Read the model definition and answer for the solid it produces. Units are mm, in the model's axes. A direction names the side the tool comes from. Coordinates: 2 decimals unless noted, no trailing zeros. Loops run counter-clockwise (first coordinate to the right, second up) from the corner with the lowest first, then second, coordinate; pieces in that order, holes last. Notation, with made-up numbers: (6, 22.25) -> (16, 22.25) arc R16 cw to (16, 48.25) -> close; hole circle Ø9 at (15.25, 2). An arc over 180 degrees is marked (long way). Answer as a JSON object with one key per item and string values. Group by question number.
1) Consider probe 1 along Y at (x, z) = (0, 1.15); probe 2 along X at (y, z) = (-7.5, 1.35); probe 3 along X at (y, z) = (-24, 2.4). Determine where each line is inside the solid, lowest interval first. Write a range as [from, to].
2) Section A-A, the plane z = 5 is taken. Count the separate pieces of the cut face and the enclosed holes in it, plus the area to 3 significant figures.
3) Determine the mould class of faces 1 (the face through (-9, 14, 3)), 2 (the face through (-13.196, 16.289, 2.958)), 3 (the face through (0, -8, 6)) for opening direction Y: released by +Y, released by -Y, zero draft, split by the parting line, or undercut.
4) Which of the six approach directions +Z, -Z, +X, -X, +Y, -Y give full straight-line access (tool end or side, diameter ignored) to faces 4 (the face through (0, -34.506, 3)), 5 (the face through (3.3, -18.4, 5)), 6 (the face through (9, 4, 3))?
5) Section D-D, the plane x = 6 is taken. Give the vertices of the cut face in (y, z).
6) Section B-B, the plane y = -9 is taken. Give the vertices of the cut face in (x, z).
7) Flat-ended cylindrical pins translate along their axes: P1, Ø4, axis at x = -2, y = -24.5, coming from the +Z side; P2, Ø1.6, axis at y = -25, z = 4.5, coming from the -X side. Find the tip coordinate at first contact, or state that the pin passes through.
from build123d import *

# Parameters (mm, degrees)
SKETCH_R     = 4
PAD_DEPTH    = 6
POCKET_DEPTH = 2


with BuildPart() as part:
    # Sketch → Pad (new body)
    with BuildSketch(Plane.XY):
        with BuildLine():
            Line((-9, 18), (9, 18))
            ThreePointArc((15, 12), (13.242641, 16.242641), (9, 18))
            Line((15, 12), (15, -24))
            ThreePointArc((4.494447, -34.505553), (11.922995, -31.428548), (15, -24))
            Line((4.494447, -34.505553), (-4.494447, -34.505553))
            ThreePointArc((-15, -24), (-11.922995, -31.428548), (-4.494447, -34.505553))
            Line((-15, -24), (-15, 12))
            ThreePointArc((-9, 18), (-13.242641, 16.242641), (-15, 12))
        make_face()
        with Locations((0, -24)):
            Circle(SKETCH_R, mode=Mode.SUBTRACT)
        with BuildLine():
            ThreePointArc((7, 6), (9, 4), (11, 6))
            Line((11, 6), (11, 12))
            ThreePointArc((11, 12), (9, 14), (7, 12))
            Line((7, 6), (7, 12))
        make_face(mode=Mode.SUBTRACT)
        with BuildLine():
            ThreePointArc((-11, 6), (-9, 4), (-7, 6))
            Line((-7, 6), (-7, 12))
            ThreePointArc((-7, 12), (-9, 14), (-11, 12))
            Line((-11, 6), (-11, 12))
        make_face(mode=Mode.SUBTRACT)
        with BuildLine():
            ThreePointArc((7, -12), (9, -14), (11, -12))
            Line((11, -12), (11, -6))
            ThreePointArc((11, -6), (9, -4), (7, -6))
            Line((7, -12), (7, -6))
        make_face(mode=Mode.SUBTRACT)
        with BuildLine():
            ThreePointArc((-11, -12), (-9, -14), (-7, -12))
            Line((-7, -12), (-7, -6))
            ThreePointArc((-7, -6), (-9, -4), (-11, -6))
            Line((-11, -12), (-11, -6))
        make_face(mode=Mode.SUBTRACT)
        with BuildLine():
            ThreePointArc((-4, -3), (0, -7), (4, -3))
            Line((4, -3), (4, 3))
            ThreePointArc((4, 3), (0, 7), (-4, 3))
            Line((-4, -3), (-4, 3))
        make_face(mode=Mode.SUBTRACT)
    extrude(amount=PAD_DEPTH)

    # Sketch001 (on Face31 of Pad) → Pocket (cut)
    with BuildSketch(Plane.XY.offset(6)):
        Polygon((6.5, -20.247223), (0, -16.494447), (-6.5, -20.247223), (-6.5, -27.752777), (0, -31.505553), (6.5, -27.752777), align=None)
    extrude(amount=-POCKET_DEPTH, mode=Mode.SUBTRACT)


solid = part.part
Determined:
{
 "1": {"probe 1": "[-34.51, -28], [-20, -7], [7, 18]", "probe 2": "[-15, -11], [-7, 7], [11, 15]", "probe 3": "[-15, -4], [4, 15]"},
 "2": {"separate pieces": "1", "enclosed holes": "6", "area": "1,120 mm²"},
 "3": {"face 1": "undercut", "face 2": "released by +Y", "face 3": "zero draft"},
 "4": {"face 4": "+Z, -Z, +X, -X, -Y", "face 5": "+Z", "face 6": "+Z, -Z"},
 "5": {"outline": "(-34.4, 0) -> (18, 0) -> (18, 6) -> (-19.96, 6) -> (-19.96, 4) -> (-28.04, 4) -> (-28.04, 6) -> (-34.4, 6) -> close"},
 "6": {"outline": "(-15, 0) -> (-11, 0) -> (-11, 6) -> (-15, 6) -> close; (-7, 0) -> (7, 0) -> (7, 6) -> (-7, 6) -> close; (11, 0) -> (15, 0) -> (15, 6) -> (11, 6) -> close"},
 "7": {"P1": "z = 4", "P2": "x = -15"}
}
